from build123d import *

# Parameters (mm, degrees)
F1_DEPTH = 0.4
F0_W     = 15
F0_H     = 42.6826924086
F2_DEPTH = 15
F3_R     = 10
F4_R     = 5


with BuildPart() as f1:
    # F0 (on Top) → F1 (new body)
    with BuildSketch(Plane.XY):
        with BuildLine():
            ThreePointArc((0, -15.2296504378), (10.6066017178, -19.62304872), (15, -30.2296504378))
            Line((15, -30.2296504378), (20, 15.9674037131))
            Line((20, 15.9674037131), (-20, 15.9674037131))
            Line((-20, 15.9674037131), (-15, -30.2296504378))
            ThreePointArc((-15, -30.2296504378), (-10.6066017178, -19.62304872), (0, -15.2296504378))
        make_face()
    extrude(amount=F1_DEPTH)

    # F0 (on Top) → F2 (join)
    with BuildSketch(Plane.XY):
        with Locations((7.5, -51.5709966421)):
            Rectangle(F0_W, F0_H)
        with BuildLine():
            Line((0, -30.2296504378), (15, -30.2296504378))
            ThreePointArc((15, -30.2296504378), (10.6066017178, -19.62304872), (0, -15.2296504378))
            Line((0, -15.2296504378), (0, -30.2296504378))
        make_face()
        with BuildLine():
            Line((-15, -30.2296504378), (0, -30.2296504378))
            Line((0, -30.2296504378), (0, -15.2296504378))
            ThreePointArc((0, -15.2296504378), (-10.6066017178, -19.62304872), (-15, -30.2296504378))
        make_face()
        with Locations((-7.5, -51.5709966421)):
            Rectangle(F0_W, F0_H)
    extrude(amount=F2_DEPTH)

    # F3
    f3_edges = [f1.edges().sort_by_distance(p)[0] for p in [
        (0, -15.22965, 15),
    ]]
    fillet(f3_edges, radius=F3_R)

    # F4
    f4_edges = [f1.edges().sort_by_distance(p)[0] for p in [
        (12.071068, -72.912343, 12.071068),
    ]]
    fillet(f4_edges, radius=F4_R)


solid = f1.part
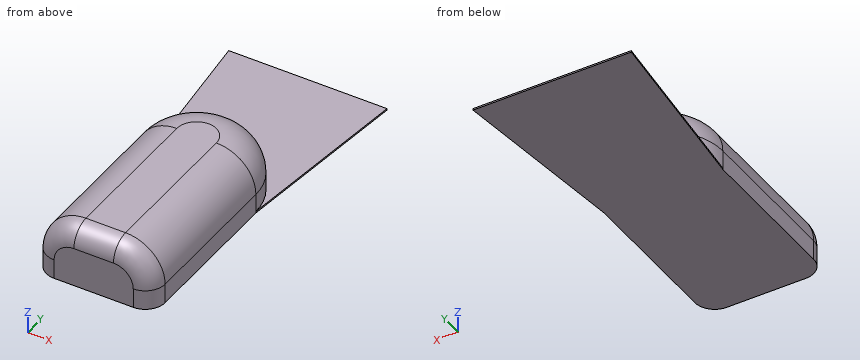
Design review of the part built by this model. Coordinates are the model's own, in mm. Round coordinates to 2 decimals unless told otherwise and drop trailing zeros. Write each loop counter-clockwise with the first axis right and the second up, starting at its lowest first coordinate (ties: lowest second). Pieces come first, ordered by that corner, then holes. Notation, with made-up numbers: (-31, 14.25) - (7, 14.25) arc R28 cw to (7, 48.25) - close; hole circle Ø9 at (66.25, 77). An arc over 180 degrees is marked (long way). Use a Markdown table: item, result. Add a question column.
1. We need section B-B (y = -37). State the section outline as (x, z) points.
2. We need section A-A (z = 1.5). State the section outline as (x, y) points, then the cut area to 3 significant figures.
3. Clearance check with flat-ended pins moving along their axes: pin 1 (1 mm diameter, centred on y = -32, z = 9.5, fed in from -X); pin 2 (3 mm diameter, centred on y = -63, z = 7.5, fed in from +X); pin 3 (2.5 mm diameter, centred on y = -49, z = 1.5, fed in from +X). State where each tip first meets the part, or that it passes through.
4. Wall thickness on probe 1 along X at (y, z) = (-51, 4.25); probe 2 along Z at (x, y) = (-5.5, 4); probe 3 along Y at (x, z) = (-3, 3): over which ranges is each line inside the solid? List them lowest first.
5. We need section C-C (y = 1). State the section outline as (x, z) points, then the cut area to 3 significant figures.
Output:
| question | item | result |
|---|---|---|
| 1 | outline | (-15, 0) - (15, 0) - (15, 5) arc R10 ccw to (5, 15) - (-5, 15) arc R10 ccw to (-15, 5) - close |
| 2 | outline | (-15, -67.91) arc R5 ccw to (-10, -72.91) - (10, -72.91) arc R5 ccw to (15, -67.91) - (15, -30.23) arc R15 ccw to (-15, -30.23) - close |
| 2 | area | 1,620 mm2 |
| 3 | pin 1 | stops at x = -14.17 |
| 3 | pin 2 | stops at x = 14.95 |
| 3 | pin 3 | stops at x = 15 |
| 4 | probe 1 | x = -15 to 15 |
| 4 | probe 2 | z = 0 to 0.4 |
| 4 | probe 3 | y = -72.91 to -15.53 |
| 5 | outline | (-18.38, 0) - (18.38, 0) - (18.38, 0.4) - (-18.38, 0.4) - close |
| 5 | area | 14.7 mm2 |
